Here's the drawing with two shaded views (mm, measured from the low corner). I have some questions. A direction names the side the tool comes from. Coordinates: 2 decimals unless noted, no trailing zeros. Order: outer loops, then holes, each group sorted by start corner. A loop starts at its lowest first (then second) coordinate and runs counter-clockwise, first axis right, second up. Notation, with made-up numbers: (64.25, 28) -> (119.25, 28) arc R30 cw to (119.25, 67) -> close; hole circle Ø1 at (-38, 58). An arc over 180 degrees is marked (long way). Answer in a Markdown table with one row per item. Add a question column.
1. On a 3-axis mill with a long thin cutter (end or side, diameter ignored), from which of +Z, -Z, +X, -X, +Y, -Y can I reach the whole of each face in a straight line? I mean the marked faces 1 and 2. Say none if no direction works.
2. Imagine slicing it at D-D on y = 28. Write out the boundary of the cut face in (x, z) (3 decimals), plus the area to 3 significant figures.
3. Will these pins go through, and if not, where does the flat tip stop? pin 1 (8 mm diameter, centred on x = 23, y = 26, fed in from +Z); pin 2 (9 mm diameter, centred on y = 9, z = 11.5, fed in from -X).
4. Imagine slicing it at C-C on x = 14.5. Write out the boundary of the cut face in (y, z).
5. Imagine slicing it at B-B on z = 24. Write out the boundary of the cut face in (x, y).
6. If I drill on line 1 along Z through (x, y) = (3.5, 22.5); line 2 along X through (y, z) = (13, 23.5), over which ranges is the centre line in solid material (lowest first)? Write a range as [from, to].
7. Imagine slicing it at A-A on y = 12.5. Write out the boundary of the cut face in (x, z), plus the area to 3 significant figures.
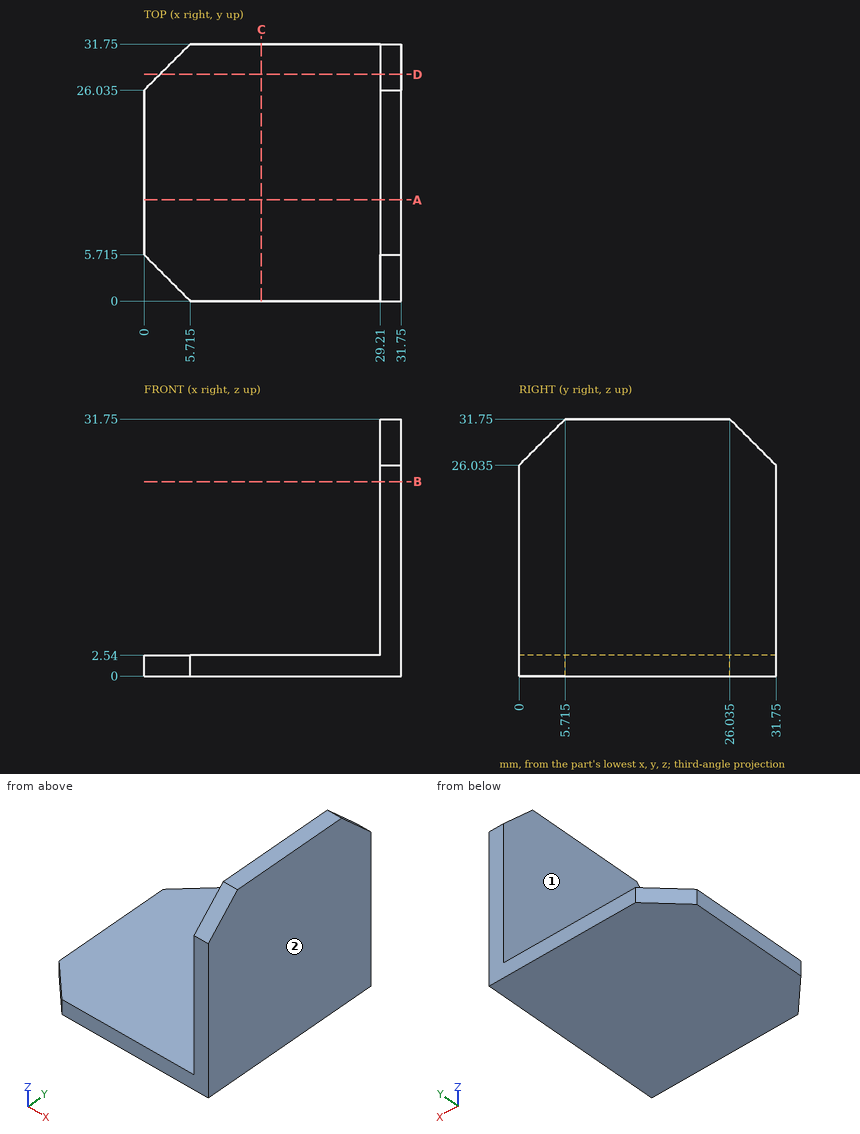
Answers follow:
| question | item | result |
|---|---|---|
| 1 | face 1 | +Z, -X, +Y, -Y |
| 1 | face 2 | +Z, -Z, +X, +Y, -Y |
| 2 | outline | (1.965, 0) -> (31.75, 0) -> (31.75, 29.785) -> (29.21, 29.785) -> (29.21, 2.54) -> (1.965, 2.54) -> close |
| 2 | area | 145 mm² |
| 3 | pin 1 | stops at z = 2.54 |
| 3 | pin 2 | stops at x = 29.21 |
| 4 | outline | (0, 0) -> (31.75, 0) -> (31.75, 2.54) -> (0, 2.54) -> close |
| 5 | outline | (29.21, 0) -> (31.75, 0) -> (31.75, 31.75) -> (29.21, 31.75) -> close |
| 6 | line 1 | z = [0, 2.54] |
| 6 | line 2 | x = [29.21, 31.75] |
| 7 | outline | (0, 0) -> (31.75, 0) -> (31.75, 31.75) -> (29.21, 31.75) -> (29.21, 2.54) -> (0, 2.54) -> close |
| 7 | area | 155 mm² |
